from build123d import *

# Parameters (mm, degrees)
SKETCH1_W           = 112
SKETCH1_H           = 70
BOSS_EXTRUDE1_DEPTH = 6
SKETCH2_R           = 1.5
CUT_EXTRUDE1_DEPTH  = 6
SKETCH3_R           = 1.5
CUT_EXTRUDE2_DEPTH  = 10


with BuildPart() as part:
    # Sketch1 → Boss-Extrude1 (new body)
    with BuildSketch(Plane(origin=(0, 0, 0), x_dir=(1, 0, 0), z_dir=(0, 1, 0))):
        with Locations((56, 35)):
            Rectangle(SKETCH1_W, SKETCH1_H)
    extrude(amount=BOSS_EXTRUDE1_DEPTH)

    # Sketch2 → Cut-Extrude1 (cut)
    with BuildSketch(Plane(origin=(0, 6, 0), x_dir=(1, 0, 0), z_dir=(0, 1, 0))):
        with Locations(Location((62.735, 51.265, 0), (0, 0, 270))):
            Circle(SKETCH2_R)
        with Locations(Location((95.265, 51.265, 0), (0, 0, 270))):
            Circle(SKETCH2_R)
        with Locations(Location((62.735, 18.735, 0), (0, 0, 270))):
            Circle(SKETCH2_R)
        with Locations(Location((95.265, 18.735, 0), (0, 0, 270))):
            Circle(SKETCH2_R)
        with Locations(Location((16.735, 18.735, 0), (0, 0, 90))):
            Circle(SKETCH2_R)
        with Locations(Location((16.735, 51.265, 0), (0, 0, 90))):
            Circle(SKETCH2_R)
        with Locations(Location((49.265, 51.265, 0), (0, 0, 90))):
            Circle(SKETCH2_R)
        with Locations(Location((49.265, 18.735, 0), (0, 0, 90))):
            Circle(SKETCH2_R)
    extrude(amount=-CUT_EXTRUDE1_DEPTH, mode=Mode.SUBTRACT)

    # Sketch3 → Cut-Extrude2 (cut)
    with BuildSketch(Plane(origin=(0, 6, 0), x_dir=(1, 0, 0), z_dir=(0, 1, 0))):
        with Locations(Location((4, 57, 0), (0, 0, 270))):
            Circle(SKETCH3_R)
        with Locations(Location((13, 66, 0), (0, 0, 270))):
            Circle(SKETCH3_R)
        with Locations(Location((99, 66, 0), (0, 0, 90))):
            Circle(SKETCH3_R)
        with Locations(Location((108, 57, 0), (0, 0, 90))):
            Circle(SKETCH3_R)
        with Locations(Location((108, 13, 0), (0, 0, 270))):
            Circle(SKETCH3_R)
        with Locations(Location((99, 4, 0), (0, 0, 270))):
            Circle(SKETCH3_R)
        with Locations(Location((13, 4, 0), (0, 0, 90))):
            Circle(SKETCH3_R)
        with Locations(Location((4, 13, 0), (0, 0, 90))):
            Circle(SKETCH3_R)
    extrude(amount=-CUT_EXTRUDE2_DEPTH, mode=Mode.SUBTRACT)


solid = part.part
The model under review builds one solid part; all positions refer to its coordinate system, in mm. Give positions to 0.01 mm unless a question says otherwise; leave off trailing zeros. Write each loop counter-clockwise with the first axis right and the second up, starting at its lowest first coordinate (ties: lowest second). Pieces come first, ordered by that corner, then holes.
1. Wall thickness on L1, parallel to X at y = 2.1, z = -66; L2, parallel to X at y = 3.5, z = -13; L3, parallel to Z at x = 99, y = 4: over which ranges is each line inside the solid? List them lowest first.
2. Add section A-A, the plane x = 4. Write out the cut boundary in (y, z), plus the area to 3 significant figures.
3. Add section B-B, the plane z = -57. Write out the cut boundary in (x, y).
4. Draft analysis for pull direction Z (two halves, no side actions). For faces 1 (the flat face through (55, 3, -70)), 2 (the cylindrical face through (106.735, 3.042, -57.806)), 3 (the flat face through (0, 3, -35)), 4 (the flat face through (55, 3, 0)), state which applies: +Z half, -Z half, draft (parallel to the pull), parting line (faces both ways), or undercut.
Worked answers:
1. L1: x = 0 to 11.5, 14.5 to 97.5, 100.5 to 112
1. L2: x = 0 to 2.5, 5.5 to 106.5, 109.5 to 112
1. L3: z = -70 to -67.5, -64.5 to -5.5, -2.5 to 0
2. outline: (0, -70) - (6, -70) - (6, -58.5) - (0, -58.5) - close; (0, -55.5) - (6, -55.5) - (6, -14.5) - (0, -14.5) - close; (0, -11.5) - (6, -11.5) - (6, 0) - (0, 0) - close
2. area: 384 mm2
3. outline: (0, 0) - (2.5, 0) - (2.5, 6) - (0, 6) - close; (5.5, 0) - (106.5, 0) - (106.5, 6) - (5.5, 6) - close; (109.5, 0) - (112, 0) - (112, 6) - (109.5, 6) - close
4. face 1: -Z half
4. face 2: undercut
4. face 3: draft
4. face 4: +Z half
